Source: CAD feature listing. Evaluate the final solid. Frame: model axes, mm. Face numbers are marked on the shaded views. A direction names the side the tool comes from. Round coordinates to 2 decimals unless told otherwise and drop trailing zeros. Loops run counter-clockwise (first coordinate to the right, second up) from the corner with the lowest first, then second, coordinate; pieces in that order, holes last. Notation, with made-up numbers: (31, 79) - (44, 79) arc R23 ccw to (44, 93) - close; hole circle Ø6 at (65, 85). An arc over 180 degrees is marked (long way). One line per question, with ' | ' between items. Start each with the question number.
1. Ray query, line 1 (X direction, y = -36.25, z = 0); line 2 (Y direction, x = -20.5, z = -4.5); line 3 (X direction, y = -1.8, z = 0). Return the intervals inside material, ascending.
2. Cut plane A-A (x = -20). Return loops of the section in (y, z), then the cut area to 3 significant figures.
3. Access query for the marked faces 1, 2 and 3. Directions: +Z, -Z, +X, -X, +Y, -Y. A direction counts if a zero-diameter tool reaches every point of the face in a straight line with its end or side. Return the directions, or none.
4. Cut plane B-B (z = -1.5). State how many separate pieces and enclosed holes the cut face has, then the cut area to 3 significant figures.
5. Cut plane D-D (z = 4). Return loops of the section in (x, y), then the cut area to 3 significant figures.
6. Cut plane C-C (y = -35). Return loops of the section in (x, z), then the cut area to 3 significant figures.
7. Mould query, pull axis Y, two halves, no side actions, for the marked faces 4, 5, 6 and 7. Classes: pulls with the +Y half, pulls with the -Y half, needs draft (parallel to the pull), parting line crosses it, or undercut.
8. Pin query (flat end, axial travel): pin 1 (1.5 mm diameter, centred on x = 2, z = 4, fed in from +Y); pin 2 (1 mm diameter, centred on x = 6.5, z = -1.5, fed in from +Y); pin 3 (3 mm diameter, centred on y = -12.5, z = -0.5, fed in from +X); pin 4 (5 mm diameter, centred on x = -10, z = -1.5, fed in from +Y). Return the tip coordinate at first contact, or that it passes through.
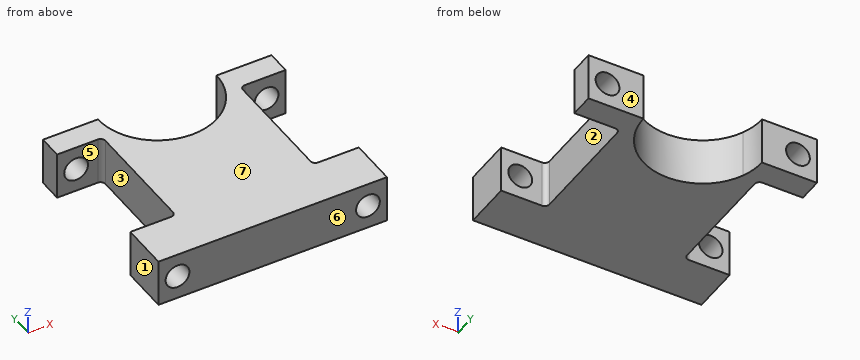
```python
from build123d import *

# Parameters (mm, degrees)
EXTRUDE_1_DEPTH     = 5
SKETCH_3_W          = 48
SKETCH_3_H          = 10
SKETCH_3_R          = 2.5
EXTRUDE_2_DEPTH     = 10
EXTRUDE_START       = -5
SKETCH_4_W          = 48
SKETCH_4_H          = 10
SKETCH_4_R          = 2.5
EXTRUDE_3_DEPTH     = 5
SKETCH_5_W          = 2
SKETCH_5_H          = 26
EXTRUDE_4_DEPTH     = 10
SKETCH_6_R          = 12.45
CUT_EXTRUDE_1_DEPTH = 16
FILLET_2_R          = 1
FILLET_3_R          = 1


with BuildPart() as part:
    # 草图1 → 凸台-拉伸1 (new, symmetric)
    with BuildSketch(Plane.XY):
        with BuildLine():
            Line((12.45, 0), (12.45, -41))
            Line((12.45, -41), (-12.45, -41))
            Line((-12.45, -41), (-12.45, 0))
            ThreePointArc((-12.45, 0), (0, -12.45), (12.45, 0))
        make_face()
    extrude(amount=EXTRUDE_1_DEPTH, both=True)

    # 草图3 → 凸台-拉伸2 (add)
    with BuildSketch(Plane.XZ.offset(41)):
        Rectangle(SKETCH_3_W, SKETCH_3_H)
        with Locations(Location((20, 0, 0), (0, 0, 270))):
            Circle(SKETCH_3_R, mode=Mode.SUBTRACT)
        with Locations(Location((-20, 0, 0), (0, 0, 90))):
            Circle(SKETCH_3_R, mode=Mode.SUBTRACT)
    extrude(amount=-EXTRUDE_2_DEPTH)

    # 草图4 → 凸台-拉伸3 (add)
    with BuildSketch(Plane(origin=(0, 0, 0), x_dir=(1, 0, 0), z_dir=(0, 1, 0)).offset(EXTRUDE_START)):
        Rectangle(SKETCH_4_W, SKETCH_4_H)
        with Locations(Location((-20, 0, 0), (0, 0, 270))):
            Circle(SKETCH_4_R, mode=Mode.SUBTRACT)
        with Locations(Location((20, 0, 0), (0, 0, 90))):
            Circle(SKETCH_4_R, mode=Mode.SUBTRACT)
    extrude(amount=EXTRUDE_3_DEPTH)

    # 草图5 → 凸台-拉伸4 (add)
    with BuildSketch(Plane.XY.offset(5)):
        with Locations((-13.45, -18)):
            Rectangle(SKETCH_5_W, SKETCH_5_H)
        with Locations((13.45, -18)):
            Rectangle(SKETCH_5_W, SKETCH_5_H)
    extrude(amount=-EXTRUDE_4_DEPTH)

    # 草图6 → 切除-拉伸1 (cut)
    with BuildSketch(Plane.XY.offset(5)):
        Circle(SKETCH_6_R)
    extrude(amount=-CUT_EXTRUDE_1_DEPTH, mode=Mode.SUBTRACT)

    # 圆角2
    fillet_2_edges = [part.edges().sort_by_distance(p)[0] for p in [
        (-14.45, -31, 0),
        (14.45, -31, 0),
    ]]
    fillet(fillet_2_edges, radius=FILLET_2_R)

    # 圆角3
    fillet_3_edges = [part.edges().sort_by_distance(p)[0] for p in [
        (-14.45, -5, 0),
        (14.45, -5, 0),
    ]]
    fillet(fillet_3_edges, radius=FILLET_3_R)


solid = part.part
```
Answers follow:
1) line 1: x = -24 to -22.5, -17.5 to 17.5, 22.5 to 24 | line 2: y = -41 to -31, -5 to 0 | line 3: x = -24 to -22.5, -17.5 to -12.32, 12.32 to 17.5, 22.5 to 24
2) outline: (-41, -5) - (-31, -5) - (-31, -2.5) - (-41, -2.5) - close; (-41, 2.5) - (-31, 2.5) - (-31, 5) - (-41, 5) - close; (-5, -5) - (0, -5) - (0, -2.5) - (-5, -2.5) - close; (-5, 2.5) - (0, 2.5) - (0, 5) - (-5, 5) - close | area: 75.0 mm2
3) face 1: +Z, -Z, -X, +Y, -Y | face 2: +Z, -Z, +X | face 3: +Z, -Z, -X
4) separate pieces: 5 | enclosed holes: 0 | area: 1,110 mm2
5) outline: (-24, -41) - (24, -41) - (24, -31) - (15.45, -31) arc R1 cw to (14.45, -30) - (14.45, -6) arc R1 cw to (15.45, -5) - (24, -5) - (24, 0) - (12.45, 0) arc R12.45 cw to (-12.45, 0) - (-24, 0) - (-24, -5) - (-15.45, -5) arc R1 cw to (-14.45, -6) - (-14.45, -30) arc R1 cw to (-15.45, -31) - (-24, -31) - close | area: 1,230 mm2
6) outline: (-24, -5) - (24, -5) - (24, 5) - (-24, 5) - close; hole circle Ø5 at (-20, 0); hole circle Ø5 at (20, 0) | area: 441 mm2
7) face 4: pulls with the +Y half | face 5: undercut | face 6: pulls with the -Y half | face 7: needs draft
8) pin 1: stops at y = -12.14 | pin 2: stops at y = -10.3 | pin 3: stops at x = 14.45 | pin 4: stops at y = 0
